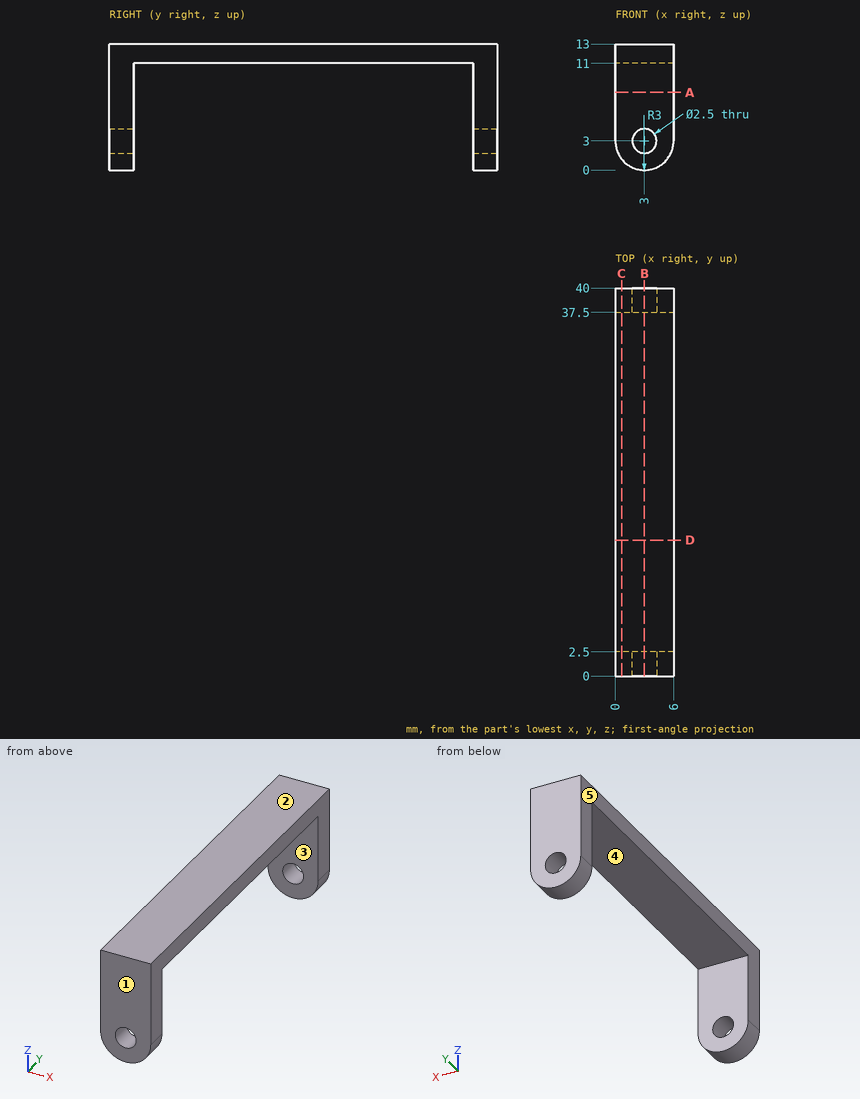
Could you check a few things on this drawing? It's one solid part, dimensions in mm from its lowest x, y, z. A direction names the side the tool comes from. Coordinates: 2 decimals unless noted, no trailing zeros. Write each loop counter-clockwise with the first axis right and the second up, starting at its lowest first coordinate (ties: lowest second). Pieces come first, ordered by that corner, then holes. Notation, with made-up numbers: (21.5, 39) - (75.5, 39) arc R31 ccw to (75.5, 71) - close; hole circle Ø3 at (69, 80). An arc over 180 degrees is marked (long way). Use one line per item in the form item = value.
1) I need wall thicknesses on line 1 (Y direction, x = 4.4, z = 4.5); line 2 (Z direction, x = 3, y = 1.25); line 3 (Z direction, x = 3.55, y = 17.5). Which ranges of each line are inside material? Lowest first, please.
Solved:
line_1 = 0 to 2.5, 37.5 to 40
line_2 = 0 to 1.75, 4.25 to 13
line_3 = 11 to 13
2) Suppose I cut it at B-B, the plane x = 3. Write out the boundary of the cut face in (y, z), plus the area to 4 significant figures.
Solved:
outline = (0, 0) - (2.5, 0) - (2.5, 1.75) - (0, 1.75) - close; (0, 4.25) - (2.5, 4.25) - (2.5, 11) - (37.5, 11) - (37.5, 4.25) - (40, 4.25) - (40, 13) - (0, 13) - close; (37.5, 0) - (40, 0) - (40, 1.75) - (37.5, 1.75) - close
area = 122.5 mm2
3) Thinking about a two-plate mould opening in Y: for the marked faces 1, 2 and 3, which applies, released by +Y, released by -Y, zero draft, split by the parting line, or undercut?
Solved:
face_1 = released by -Y
face_2 = zero draft
face_3 = undercut
4) I'm going to push a flat-ended pin straight in: P1, Ø3, axis at x = 4.5, y = 22, coming from the -Z side. Where does the tip first touch, or does it pass through?
Solved:
P1 = 11
5) Suppose I cut it at C-C, the plane x = 0.65. Write out the boundary of the cut face in (y, z).
Solved:
outline = (0, 1.14) - (2.5, 1.14) - (2.5, 11) - (37.5, 11) - (37.5, 1.14) - (40, 1.14) - (40, 13) - (0, 13) - close
6) Suppose I cut it at D-D, the plane y = 14. Write out the boundary of the cut face in (x, z), plus the area to 3 significant figures.
Solved:
outline = (0, 11) - (6, 11) - (6, 13) - (0, 13) - close
area = 12.0 mm2
7) On a 3-axis mill with a long thin cutter (end or side, diameter ignored), from which of +Z, -Z, +X, -X, +Y, -Y can I reach the whole of each face in a straight line? I mean the marked faces 4 and 5. Say none if no direction works.
Solved:
face_4 = -Z, +X, -X
face_5 = +Z, -Z, -X, +Y, -Y
8) Suppose I cut it at A-A, the plane z = 8. Write out the boundary of the cut face in (x, y), plus the area to 3 significant figures.
Solved:
outline = (0, 0) - (6, 0) - (6, 2.5) - (0, 2.5) - close; (0, 37.5) - (6, 37.5) - (6, 40) - (0, 40) - close
area = 30.0 mm2
